Geometry check sheet. Reference: the model listing, model coordinates, mm. A direction names the side the tool comes from. Round coordinates to 2 decimals unless told otherwise and drop trailing zeros. Loops run counter-clockwise (first coordinate to the right, second up) from the corner with the lowest first, then second, coordinate; pieces in that order, holes last. Notation, with made-up numbers: (54, 56) -> (109, 56) arc R20 ccw to (109, 61) -> close; hole circle Ø5 at (74, -5.75). An arc over 180 degrees is marked (long way). Use one line per item in the form item = value.
from build123d import *

# Parameters (mm, degrees)
CHAMFER1_SIZE = 0.2
CHAMFER2_SIZE = 0.2


with BuildPart() as part:
    # Sketch1 → Revolve1 (revolve)
    with BuildSketch(Plane(origin=(0, 0, 0), x_dir=(1, 0, 0), z_dir=(0, 1, 0))):
        with BuildLine():
            Line((2.45, 0), (0, 0))
            Line((0, 0), (0, 8.9))
            Line((0, 8.9), (9.75, 8.9))
            ThreePointArc((9.75, 8.9), (10.457106781, 8.607106781), (10.75, 7.9))
            Line((10.75, 7.9), (10.75, 7.3))
            Line((10.75, 7.3), (5.75, 7.3))
            Line((5.75, 7.3), (5.75, 6.9))
            Line((5.75, 6.9), (2.45, 6.9))
            Line((2.45, 6.9), (2.45, 0))
        make_face()
    revolve(axis=Axis((0, 0, 0), (0, 0, -1)))

    # Chamfer1
    chamfer1_edges = [part.edges().sort_by_distance(p)[0] for p in [
        (-5.75, 0, -6.9),
    ]]
    chamfer(chamfer1_edges, length=CHAMFER1_SIZE)

    # Chamfer2
    chamfer2_edges = [part.edges().sort_by_distance(p)[0] for p in [
        (-2.45, 0, 0),
    ]]
    chamfer(chamfer2_edges, length=CHAMFER2_SIZE)


solid = part.part
1. Section check C-C (z = -2.5). Record the boundary of the cut face in (x, y).
Return value:
outline = circle Ø4.9 at (0, 0)
2. Tool access check on faces 1 (the cylindrical face through (-1.4, -10.66, -7.6)), 2 (the flat face through (5, 5, -7.3)). Record the directions out of +Z, -Z, +X, -X, +Y, -Y that give a thin tool (end or side, any length) a straight path to the whole face; none if there is none.
Return value:
face_1 = +Z, -Z
face_2 = +Z
3. Material ranges on line 1 along Z through (x, y) = (-6.75, 1); line 2 along Z through (x, y) = (-4.5, -1); line 3 along Y through (x, z) = (0, -6.75), recorded low to high.
Return value:
line_1 = -8.9 to -7.3
line_2 = -8.9 to -6.9
line_3 = -2.45 to 2.45
4. Gauge pin test, flat ends, axial feed: pin 1 (5 mm diameter, centred on y = 3.5, z = -6, fed in from -X); pin 2 (5 mm diameter, centred on y = -3.5, z = -2.5, fed in from +X); pin 3 (4 mm diameter, centred on x = 3, z = -6, fed in from -Y). Record the tip position at first contact, or that the pin passes through.
Return value:
pin_1 = -10.66
pin_2 = 2.24
pin_3 = -10.65
5. Section check A-A (y = 0). Record the boundary of the cut face in (x, z).
Return value:
outline = (-10.75, -7.9) arc R1 ccw to (-9.75, -8.9) -> (9.75, -8.9) arc R1 ccw to (10.75, -7.9) -> (10.75, -7.3) -> (5.75, -7.3) -> (5.75, -7.1) -> (5.55, -6.9) -> (2.45, -6.9) -> (2.45, -0.2) -> (2.25, 0) -> (-2.25, 0) -> (-2.45, -0.2) -> (-2.45, -6.9) -> (-5.55, -6.9) -> (-5.75, -7.1) -> (-5.75, -7.3) -> (-10.75, -7.3) -> close
